Geometry: final body of the model. Coordinates: model frame, mm. A direction names the side the tool comes from. Give positions to 0.01 mm unless a question says otherwise; leave off trailing zeros. One line per question, with ' | ' between items. Start each with the question number.
(1) First-contact query: pin 1 Ø6.5 at (x, y) = (31.75, 31.75) entering from +Z; pin 2 Ø4.5 at (x, y) = (69.85, 31.75) entering from +Z; pin 3 Ø2.5 at (x, z) = (37, 1.5) entering from +Y; pin 4 Ø2.5 at (x, y) = (31.75, 19.05) entering from -Z. Flat tips, straight axial feed; report the tip coordinate or a pass-through.
(2) Ray query, L1, parallel to Y at x = 69.85, z = -2.95; L2, parallel to Y at x = 35.5, z = 0 (3 decimals); L3, parallel to Y at x = 10, z = 1.5 (3 decimals). Return the intervals inside material, ascending.
(3) Mould query, pull axis X, two halves, no side actions, for faces 1 (the face through (75.436, 0.724, -2.828)), 2 (the face through (68.18, 5.28, -3.57)), 3 (the face through (38, 50.8, -3)). Classes: +X half, -X half, draft (parallel to the pull), parting line (faces both ways), or undercut.
(4) Set-up query: faces 4 (the face through (72.857, 7.37, 0.634)), 5 (the face through (30.409, 45.913, -3.57)). Return all of +Z, -Z, +X, -X, +Y, -Y with unobstructed straight access to the full face (end or side cutting, diameter ignored); none if empty.
(5) Section A-A (z = -3). State how many separate pieces and enclosed holes the cut face has, then the cut area to 3 significant figures.
```python
from build123d import *

# Parameters (mm, degrees)
BOSS_EXTRUDE1_DEPTH             = 76.2
FILLET1_R                       = 2.54
CUT_EXTRUDE1_DEPTH              = 5.08
F_5_32_0_15625_DIAMETER_HOLE1_D = 3.96875


with BuildPart() as part:
    # Sketch3 → Boss-Extrude1 (new body)
    with BuildSketch(Plane(origin=(0, 0, 0), x_dir=(0, 0, -1), z_dir=(1, 0, 0))):
        with BuildLine():
            ThreePointArc((-0.5955037838105575, 1.7517241379310349), (-0.3542263859949928, 1.225338953378048), (-1.2301e-13, 0.7672780265587602))
            Line((0, 0.7672780265588011), (0, 50.0327219734412))
            ThreePointArc((-1.2323e-13, 50.03272197344124), (-0.3542263859949948, 49.57466104662194), (-0.5955037838105568, 49.04827586206895))
            ThreePointArc((-0.5955037838105568, 49.04827586206895), (-4.35795103144676, 25.399999999999988), (-0.5955037838105568, 1.7517241379310349))
        make_face()
        with BuildLine():
            Line((0, 50.0327219734412), (0, 0.7672780265588011))
            ThreePointArc((-1.2301e-13, 0.7672780265587602), (0.8319424657603935, 0.19966735136426017), (1.8190813079349, -4.4e-16))
            Line((1.8190813079349, 0), (3.8099999999999925, 0))
            ThreePointArc((3.8099999999999925, 4.4e-16), (5.606051224213842, 0.7439487757861691), (6.350000000000011, 2.5400000000000182))
            Line((6.350000000000011, 2.5400000000000205), (6.3500000000000005, 48.26))
            ThreePointArc((6.350000000000003, 48.26), (5.606051224213832, 50.05605122421383), (3.81, 50.8))
            Line((3.8100000000000005, 50.8), (1.8190813079348995, 50.8))
            ThreePointArc((1.8190813079348995, 50.8), (0.8319424657603925, 50.60033264863574), (-1.2323e-13, 50.03272197344124))
        make_face()
    extrude(amount=BOSS_EXTRUDE1_DEPTH)

    # Fillet1
    fillet1_edges = [part.edges().sort_by_distance(p)[0] for p in [
        (0, 50.315945122036965, -0.3275419503675465),
        (0, 50.8, -2.81454065396745),
        (76.2, 0, -2.8145406539674465),
        (0, 50.05605122421383, -5.606051224213833),
        (0, 25.40000000000001, -6.350000000000006),
        (0, 0.7439487757861691, -5.606051224213842),
        (0, 0, -2.8145406539674465),
        (0, 0.4840548779630356, -0.32754195036755385),
        (76.2, 0.7439487757861691, -5.606051224213842),
        (76.2, 25.40000000000001, -6.350000000000006),
        (76.2, 50.05605122421383, -5.606051224213833),
        (76.2, 50.8, -2.81454065396745),
        (76.2, 50.31594512203697, -0.3275419503675483),
        (76.2, 25.399999999999988, 4.35795103144676),
        (76.2, 0.48405487796303426, -0.32754195036755385),
        (0, 25.399999999999988, 4.35795103144676),
    ]]
    fillet(fillet1_edges, radius=FILLET1_R)

    # Sketch5 → Cut-Extrude1 (cut)
    with BuildSketch(Plane(origin=(0, -9.9e-16, 4.368799999999987), x_dir=(-1, 0, 0), z_dir=(0, 2.3e-16, -1))):
        with BuildLine():
            Line((-6.3500000000000085, 47.625), (-69.85000000000002, 47.62499999999999))
            ThreePointArc((-69.85000000000002, 47.62499999999999), (-73.02500000000002, 44.449999999999996), (-69.85000000000002, 41.275))
            Line((-69.85000000000002, 41.275), (-6.3500000000000085, 41.275))
            ThreePointArc((-6.3500000000000085, 41.275), (-3.1750000000000114, 44.449999999999996), (-6.3500000000000085, 47.625))
        make_face()
        with BuildLine():
            Line((-6.34999999999987, 34.925), (-69.84999999999988, 34.925))
            ThreePointArc((-69.84999999999988, 34.925), (-73.02499999999988, 31.75), (-69.84999999999988, 28.575000000000003))
            Line((-69.84999999999988, 28.575000000000003), (-6.34999999999987, 28.575000000000003))
            ThreePointArc((-6.34999999999987, 28.575000000000003), (-3.174999999999873, 31.75), (-6.34999999999987, 34.925))
        make_face()
        with BuildLine():
            Line((-6.34999999999987, 15.875000000000014), (-69.84999999999988, 15.875000000000014))
            ThreePointArc((-69.84999999999988, 15.875000000000014), (-73.02499999999974, 19.049999999999997), (-69.84999999999988, 22.22500000000001))
            Line((-69.84999999999988, 22.22500000000001), (-6.34999999999987, 22.22500000000001))
            ThreePointArc((-6.34999999999987, 22.22500000000001), (-3.174999999999873, 19.05000000000001), (-6.34999999999987, 15.875000000000014))
        make_face()
        with BuildLine():
            Line((-6.3500000000000085, 3.1750000000000114), (-69.85000000000002, 3.175000000000018))
            ThreePointArc((-69.85000000000002, 3.175000000000018), (-73.02500000000002, 6.350000000000016), (-69.85000000000002, 9.525000000000013))
            Line((-69.85000000000002, 9.525000000000013), (-6.3500000000000085, 9.525000000000013))
            ThreePointArc((-6.3500000000000085, 9.525000000000013), (-3.1750000000000114, 6.350000000000016), (-6.3500000000000085, 3.1750000000000114))
        make_face()
    extrude(amount=CUT_EXTRUDE1_DEPTH, mode=Mode.SUBTRACT)

    # 5/32 (0.15625) Diameter Hole1 (through all)
    with Locations(Plane(origin=(6.35, 44.45, -0.7112), x_dir=(0, 1, 0), z_dir=(0, 0, 1))):
        with Locations((0, 0), (0, -12.7), (0, -25.4), (0, -38.1), (0, -50.8), (0, -63.5), (-12.7, 0), (-12.7, -12.7), (-12.7, -25.4), (-12.7, -38.1), (-12.7, -50.8), (-12.7, -63.5), (-25.4, -63.5), (-25.4, -50.8), (-25.4, -38.1), (-25.4, -25.4), (-25.4, -12.7), (-25.4, 0), (-38.1, 0), (-38.1, -12.7), (-38.1, -25.4), (-38.1, -38.1), (-38.1, -50.8), (-38.1, -63.5)):
            Hole(F_5_32_0_15625_DIAMETER_HOLE1_D / 2)


solid = part.part
```
Response:
1) pin 1: stops at z = 4.29 | pin 2: stops at z = -0.71 | pin 3: stops at y = 49.73 | pin 4: passes through
2) L1: y = 0 to 4.37, 8.33 to 17.07, 21.03 to 29.77, 33.73 to 42.47, 46.43 to 50.8 | L2: y = 0.767 to 3.175, 9.525 to 15.875, 22.225 to 28.575, 34.925 to 41.275, 47.625 to 50.033 | L3: y = 9.525 to 15.875, 22.225 to 28.575, 34.925 to 41.275
3) face 1: +X half | face 2: undercut | face 3: draft
4) face 4: +Z | face 5: +Z, -Z
5) separate pieces: 1 | enclosed holes: 24 | area: 3,570 mm^2
